CAD build for the part. Positions are in the model's coordinates, mm. Face numbers are marked on the shaded views. Round coordinates to 2 decimals unless told otherwise and drop trailing zeros. Loops run counter-clockwise (first coordinate to the right, second up) from the corner with the lowest first, then second, coordinate; pieces in that order, holes last. Notation, with made-up numbers: M 70.5,87.5 L 123.5,87.5 A16 ccw 123.5,91.5 Z; hole C -25,-23.5 d10. An arc over 180 degrees is marked long. Use a Markdown table: item, result. Add a question column.
(1) Two-plate mould, pull along Y, no slides. Class the marked faces 1, 2 and 3: released by +Y, released by -Y, zero draft, split by the parting line, or undercut.
(2) Band-saw the part on D-D, the plane y = 0. Write the cut outline in (x, z), and give its area (3 significant figures).
(3) Band-saw the part on C-C, the plane x = 9. Write the cut outline in (y, z), and give its area (3 significant figures).
(4) Flat gauge pins, fed straight in: P1, Ø1.5, axis at x = 1.5, y = -0.5, coming from the -Z side; P2, Ø3, axis at x = 5, z = 2.5, coming from the -Y side; P3, Ø2, axis at x = 7, z = 7, coming from the -Y side. Where does each tip first touch, or does it go through?
(5) Wall check: L1, parallel to Y at x = 0, z = 2.5; L2, parallel to Y at x = 0, z = 6.5; L3, parallel to X at y = -25.4, z = 8.5. Give the ranges that are in metal, low to high.
(6) Band-saw the part on A-A, the plane z = 7. Give the number of separate pieces and of enclosed holes in the cut face, and give its area (3 significant figures).
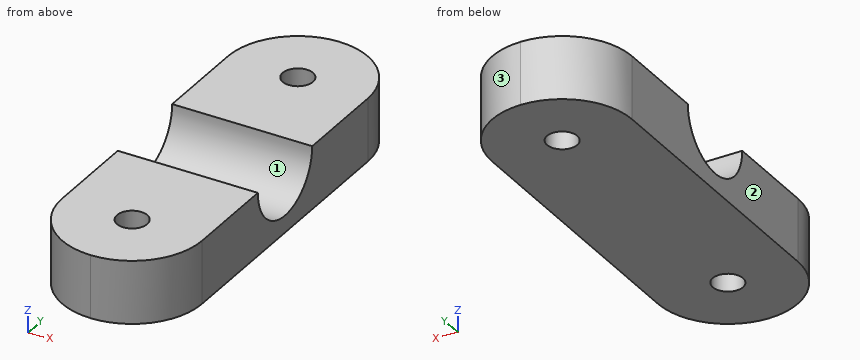
from build123d import *

# Parameters (mm, degrees)
F0_W          = 25.4
F0_H          = 76.2
F1_DEPTH      = 11.43
F3_DEPTH      = 12.701
F3_DEPTH_BACK = 12.701
F5_D          = 5.5
F6_R          = 12.69999


# Not quite as in the source:
# - a fillet or chamfer is up to 0.001 mm smaller than in the source, because OpenCascade refuses the exact size
# - a pattern or mirror of a feature is missing from the dataset's text; its kind, count and spacing are read off the source's solid


with BuildPart() as f1:
    # F0 (on Top) → F1 (new body)
    with BuildSketch(Plane.XY):
        Rectangle(F0_W, F0_H)
    extrude(amount=F1_DEPTH)

    # F2 (on Right) → F3 (cut, two sides)
    with BuildSketch(Plane.YZ) as f3_sk:
        with BuildLine():
            Line((8.334375, 11.43), (-8.334375, 11.43))
            ThreePointArc((-8.334375, 11.43), (0, 3.095625), (8.334375, 11.43))
        make_face()
    extrude(amount=-F3_DEPTH, mode=Mode.SUBTRACT)
    extrude(f3_sk.sketch, amount=F3_DEPTH_BACK, mode=Mode.SUBTRACT)

    # F5 (through all)
    with Locations(Plane(origin=(0, 0, 0), x_dir=(1, 0, 0), z_dir=(0, 0, -1))):
        with Locations((0, 25.4)):
            f5 = Hole(F5_D / 2)

    # F5_copies: F5 across plane
    add(f5.mirror(Plane.ZX), mode=Mode.SUBTRACT)

    # F6 (radius 12.7 in the source; OpenCascade refuses exactly that, so slightly less here)
    f6_edges = [f1.edges().sort_by_distance(p)[0] for p in [
        (-12.7, -38.1, 5.715),
        (12.7, -38.1, 5.715),
        (-12.7, 38.1, 5.715),
        (12.7, 38.1, 5.715),
    ]]
    fillet(f6_edges, radius=F6_R)


solid = f1.part
Return value:
| question | item | result |
|---|---|---|
| 1 | face 1 | undercut |
| 1 | face 2 | zero draft |
| 1 | face 3 | released by +Y |
| 2 | outline | M -12.7,0 L 12.7,0 L 12.7,3.1 L -12.7,3.1 Z |
| 2 | area | 78.6 mm^2 |
| 3 | outline | M -34.36,0 L 34.36,0 L 34.36,11.43 L 8.33,11.43 A8.33 cw -8.33,11.43 L -34.36,11.43 Z |
| 3 | area | 676 mm^2 |
| 4 | P1 | z = 0 |
| 4 | P2 | y = -37.61 |
| 4 | P3 | y = -36.59 |
| 5 | L1 | -38.1 to -28.15, -22.65 to 22.65, 28.15 to 38.1 |
| 5 | L2 | -38.1 to -28.15, -22.65 to -6.72, 6.72 to 22.65, 28.15 to 38.1 |
| 5 | L3 | -12.7 to -2.75, 2.75 to 12.7 |
| 6 | separate pieces | 2 |
| 6 | enclosed holes | 2 |
| 6 | area | 1,390 mm^2 |
